```python
from build123d import *

# Parameters (mm, degrees)
SKETCH1_W               = 39
SKETCH1_H               = 51
BOSS_EXTRUDE1_DEPTH     = 1
SKETCH2_R               = 1.5
CUT_EXTRUDE1_DEPTH      = 33.116973706
FILLET1_R               = 2
SKETCH3_W               = 15
SKETCH3_H               = 19
BOSS_EXTRUDE2_DEPTH     = 15.5
SKETCH4_W               = 15
SKETCH4_H               = 7.5
BOSS_EXTRUDE3_DEPTH     = 10
CUT_EXTRUDE2_DEPTH      = 36.647580563
CUT_EXTRUDE2_DEPTH_BACK = 36.647580563
SKETCH6_W               = 7.62
SKETCH6_H               = 2.54
SKETCH6_W_2             = 10.16
BOSS_EXTRUDE4_DEPTH     = 2
SKETCH7_W               = 0.5
SKETCH7_H               = 0.5
BOSS_EXTRUDE5_DEPTH     = 6


with BuildPart() as part:
    # Sketch1 → Boss-Extrude1 (new body)
    with BuildSketch(Plane(origin=(0, 0, 0), x_dir=(1, 0, 0), z_dir=(0, 1, 0))):
        Rectangle(SKETCH1_W, SKETCH1_H)
    extrude(amount=BOSS_EXTRUDE1_DEPTH)

    # Sketch2 → Cut-Extrude1 (cut, through all)
    with BuildSketch(Plane(origin=(0, 1, 0), x_dir=(1, 0, 0), z_dir=(0, 1, 0))):
        with Locations(Location((-17, 22.5, 0), (0, 0, 270))):
            Circle(SKETCH2_R)
        with Locations(Location((17, 22.5, 0), (0, 0, 90))):
            Circle(SKETCH2_R)
        with Locations(Location((17, -22.5, 0), (0, 0, 270))):
            Circle(SKETCH2_R)
        with Locations(Location((-17, -22.5, 0), (0, 0, 90))):
            Circle(SKETCH2_R)
    extrude(amount=-CUT_EXTRUDE1_DEPTH, mode=Mode.SUBTRACT)

    # Fillet1
    fillet1_edges = [part.edges().sort_by_distance(p)[0] for p in [
        (19.5, 0.5, 25.5),
        (-19.5, 0.5, 25.5),
        (-19.5, 0.5, -25.5),
        (19.5, 0.5, -25.5),
    ]]
    fillet(fillet1_edges, radius=FILLET1_R)

    # Sketch3 → Boss-Extrude2 (add)
    with BuildSketch(Plane.XZ):
        with Locations((-8, 4)):
            Rectangle(SKETCH3_W, SKETCH3_H)
        with Locations((8, 4)):
            Rectangle(SKETCH3_W, SKETCH3_H)
    extrude(amount=BOSS_EXTRUDE2_DEPTH)

    # Sketch4 → Boss-Extrude3 (add)
    with BuildSketch(Plane.XZ):
        with Locations((-8, 17.45)):
            Rectangle(SKETCH4_W, SKETCH4_H)
        with Locations((8, 17.45)):
            Rectangle(SKETCH4_W, SKETCH4_H)
    extrude(amount=BOSS_EXTRUDE3_DEPTH)

    # Sketch5 → Cut-Extrude2 (cut, two sides: drawn at the far end of the back side and taken through both)
    with BuildSketch(Plane(origin=(0, 0, 0), x_dir=(0, 0, -1), z_dir=(1, 0, 0)).offset(-CUT_EXTRUDE2_DEPTH_BACK)):
        Polygon((-21.2, -10), (-21.2, -6.5), (-20.2, -10), align=None)
        Polygon((-14.7, -10), (-13.7, -10), (-13.7, -6.5), align=None)
    extrude(amount=CUT_EXTRUDE2_DEPTH + CUT_EXTRUDE2_DEPTH_BACK, mode=Mode.SUBTRACT)

    # Sketch6 → Boss-Extrude4 (add)
    with BuildSketch(Plane.XZ):
        with Locations((-7.69, -22.23)):
            Rectangle(SKETCH6_W, SKETCH6_H)
        with Locations((6.42, -22.23)):
            Rectangle(SKETCH6_W_2, SKETCH6_H)
    extrude(amount=BOSS_EXTRUDE4_DEPTH)

    # Sketch7 → Boss-Extrude5 (add)
    with BuildSketch(Plane.XZ.offset(2)):
        with Locations((7.69, -22.23)):
            Rectangle(SKETCH7_W, SKETCH7_H)
        with Locations((10.23, -22.23)):
            Rectangle(SKETCH7_W, SKETCH7_H)
        with Locations((5.15, -22.23)):
            Rectangle(SKETCH7_W, SKETCH7_H)
        with Locations((2.61, -22.23)):
            Rectangle(SKETCH7_W, SKETCH7_H)
        with Locations((-5.15, -22.23)):
            Rectangle(SKETCH7_W, SKETCH7_H)
        with Locations((-7.69, -22.23)):
            Rectangle(SKETCH7_W, SKETCH7_H)
        with Locations((-10.23, -22.23)):
            Rectangle(SKETCH7_W, SKETCH7_H)
    extrude(amount=BOSS_EXTRUDE5_DEPTH)


solid = part.part
```
Geometry check sheet. Reference: the model listing, model coordinates, mm. A direction names the side the tool comes from. Coordinates: 2 decimals unless noted, no trailing zeros. Order: outer loops, then holes, each group sorted by start corner. A loop starts at its lowest first (then second) coordinate and runs counter-clockwise, first axis right, second up. Notation, with made-up numbers: (-37.5, 48.5) - (13.5, 48.5) arc R9 ccw to (13.5, 62.5) - close; hole circle Ø2 at (-13, 9). An arc over 180 degrees is marked (long way). Answer as a JSON object with one key per item and string values. Group by question number.
Item 1: Sectioned sample at D-D, the plane y = -4.75. Give the number of separate pieces and of enclosed holes in the cut face, and give its area (3 significant figures).
Item 2: Sectioned sample at C-C, the plane x = 8.5. Record the cut outline in (y, z), and give its area (3 significant figures).
Item 3: Depth check by flat-ended pin: pin 1 Ø1.5 at (x, y) = (6.5, -1) entering from -Z; pin 2 Ø3 at (x, y) = (6.5, -11.5) entering from -Z; pin 3 Ø1 at (y, z) = (-4.5, -3.5) entering from +X. Enter the tip coordinate at first touch or a pass-through.
Item 4: Tool access check on faces 1 (the face through (8, -10, 17)), 2 (the face through (6, -1, -20.96)), 3 (the face through (-15.5, -5, 17)). Record the directions out of +Z, -Z, +X, -X, +Y, -Y that give a thin tool (end or side, any length) a straight path to the whole face; none if there is none.
Item 5: Scan lines: probe 1 along X at (y, z) = (0.8, 22.5); probe 2 along X at (y, z) = (-8, 13); probe 3 along Z at (x, y) = (8.5, -4.75). Record each from-to range of solid material in increasing order.
Item 6: Sectioned sample at A-A, the plane z = 22.5. Record the cut outline in (x, y).
Item 7: Sectioned sample at B-B, the plane y = -13.5. Record the cut outline in (x, z).
Resolved:
{
 "1": {"separate pieces": "11", "enclosed holes": "0", "area": "797 mm^2"},
 "2": {"outline": "(-15.5, -5.5) - (0, -5.5) - (0, -20.96) - (-2, -20.96) - (-2, -23.5) - (0, -23.5) - (0, -25.5) - (1, -25.5) - (1, 25.5) - (0, 25.5) - (0, 21.2) - (-6.5, 21.2) - (-10, 20.2) - (-10, 14.7) - (-6.5, 13.7) - (0, 13.7) - (0, 13.5) - (-15.5, 13.5) - close", "area": "422 mm^2"},
 "3": {"pin 1": "z = -23.5", "pin 2": "z = -5.5", "pin 3": "x = 15.5"},
 "4": {"face 1": "+Z, +X, -X, -Y", "face 2": "+X, -X, -Y", "face 3": "+Z, -Z, -X, -Y"},
 "5": {"probe 1": "-19.5 to -18.5, -15.5 to 15.5, 18.5 to 19.5", "probe 2": "-15.5 to -0.5, 0.5 to 15.5", "probe 3": "-5.5 to 13.5, 13.7 to 21.2"},
 "6": {"outline": "(-19.5, 0) - (-18.5, 0) - (-18.5, 1) - (-19.5, 1) - close; (-15.5, 0) - (15.5, 0) - (15.5, 1) - (-15.5, 1) - close; (18.5, 0) - (19.5, 0) - (19.5, 1) - (18.5, 1) - close"},
 "7": {"outline": "(-15.5, -5.5) - (-0.5, -5.5) - (-0.5, 13.5) - (-15.5, 13.5) - close; (0.5, -5.5) - (15.5, -5.5) - (15.5, 13.5) - (0.5, 13.5) - close"}
}
